The listing builds one solid part. Answer for the finished solid, in the listing's coordinates (mm). Give positions to 0.01 mm unless a question says otherwise; leave off trailing zeros. Order: outer loops, then holes, each group sorted by start corner. A loop starts at its lowest first (then second) coordinate and runs counter-clockwise, first axis right, second up. Notation, with made-up numbers: (13.5, 11) - (43.5, 11) arc R23 cw to (43.5, 47) - close; hole circle Ø8 at (59, -10). An arc over 180 degrees is marked (long way). Write each question's results on one line, items separated by ' | '. Start each with the question number.
1. Section D-D (y = 57) is taken. Give the vertices of the cut face in (x, z).
2. Section A-A (x = 46) is taken. Give the vertices of the cut face in (y, z).
3. Find the intervals of material crossed by L1, parallel to X at y = 65, z = 0.75; L2, parallel to X at y = 121, z = 0.85, in increasing order.
4. Section B-B (y = 117) is taken. Give the vertices of the cut face in (x, z).
5. Section C-C (x = 29) is taken. Give the vertices of the cut face in (y, z), and give its area (3 significant figures).
from build123d import *

# Parameters (mm, degrees)
BOSS_EXTRUDE1_DEPTH = 3
CHAMFER7_SIZE       = 1.5
CHAMFER7_SIZE_2     = 2.598076211


with BuildPart() as part:
    # Sketch1 → Boss-Extrude1 (new body)
    with BuildSketch(Plane.XY):
        Polygon((90.5, 0), (90.5, 40), (10.5, 127), (0, 127), (0, 0), align=None)
    extrude(amount=BOSS_EXTRUDE1_DEPTH)

    # Chamfer7
    # the kernel refuses this chamfer: 2.598076211, 1.5 mm, written as the material it takes off along each edge
    with BuildSketch(Plane(origin=(-6.721445956, 0, 3), x_dir=(0, -0.0578938624026714, -0.9983227437537926), z_dir=(1, 0, 0))) as chamfer7_piece_1:
        Polygon((CHAMFER7_SIZE * 0.998322743754, CHAMFER7_SIZE * 0.0578938624027), (-CHAMFER7_SIZE_2 * 0.0578938624105, CHAMFER7_SIZE_2 * 0.99832274389), (0, 0), align=None)
    extrude(amount=103.942891912, mode=Mode.SUBTRACT)
    with BuildSketch(Plane(origin=(-6.721445956, 0, 0), x_dir=(0, -0.0578938624026714, 0.9983227437537926), z_dir=(1, 0, 0))) as chamfer7_piece_2:
        Polygon((CHAMFER7_SIZE * 0.998322743754, -CHAMFER7_SIZE * 0.0578938624027), (-CHAMFER7_SIZE_2 * 0.0578938624105, -CHAMFER7_SIZE_2 * 0.99832274389), (0, 0), align=None)
    extrude(amount=103.942891912, mode=Mode.SUBTRACT)
    with BuildSketch(Plane(origin=(95.04956673, 35.052346181, 3), x_dir=(0.042615650155104184, 0.03918680474032571, -0.9983227437537929), z_dir=(-0.6768732144311417, 0.7360996206938663, 0))) as chamfer7_piece_3:
        Polygon((CHAMFER7_SIZE * 0.998322743754, CHAMFER7_SIZE * 0.0578938624027), (-CHAMFER7_SIZE_2 * 0.0578938624105, CHAMFER7_SIZE_2 * 0.99832274389), (0, 0), align=None)
    extrude(amount=131.633416067, mode=Mode.SUBTRACT)
    with BuildSketch(Plane(origin=(95.04956673, 35.052346181, 0), x_dir=(0.042615650155104184, 0.03918680474032571, 0.9983227437537929), z_dir=(-0.6768732144311417, 0.7360996206938663, 0))) as chamfer7_piece_4:
        Polygon((CHAMFER7_SIZE * 0.998322743754, -CHAMFER7_SIZE * 0.0578938624027), (-CHAMFER7_SIZE_2 * 0.0578938624105, -CHAMFER7_SIZE_2 * 0.99832274389), (0, 0), align=None)
    extrude(amount=131.633416067, mode=Mode.SUBTRACT)


solid = part.part
Reported:
1) outline: (0, 0) - (71.34, 0) - (74.87, 1.5) - (71.34, 3) - (0, 3) - close
2) outline: (0, 1.5) - (2.6, 0) - (84.56, 0) - (88.39, 1.5) - (84.56, 3) - (2.6, 3) - close
3) L1: 0 to 65.75 | L2: 0 to 14.49
4) outline: (0, 0) - (16.17, 0) - (19.7, 1.5) - (16.17, 3) - (0, 3) - close
5) outline: (0, 1.5) - (2.6, 0) - (103.04, 0) - (106.88, 1.5) - (103.04, 3) - (2.6, 3) - close | area: 311 mm²
